Study the drawing (mm; zero at the part's minimum x, y, z) and answer. Coordinates: 2 decimals unless noted, no trailing zeros. Order: outer loops, then holes, each group sorted by start corner. A loop starts at its lowest first (then second) coordinate and runs counter-clockwise, first axis right, second up.
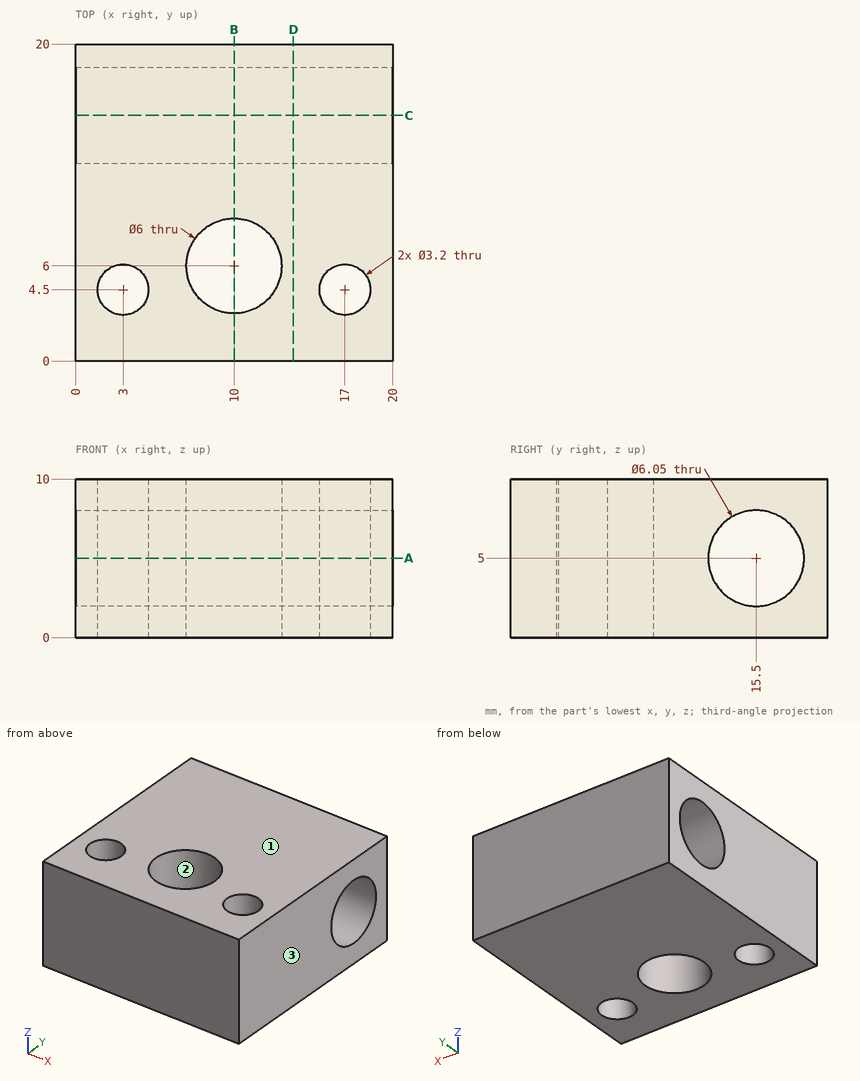
1) A flat-ended cylindrical pin translates along its axis: pin 1 Ø4 at (x, z) = (11.5, 4.5) entering from -Y. Find the tip coordinate at first contact, or state that the pin passes through.
A:
pin 1: stops at y = 0
2) A cutting plane is placed at A-A, the plane z = 5. Determine the outline of the cut face in (x, y) (3 decimals), and give its area (3 significant figures).
A:
outline: (0, 0) - (20, 0) - (20, 12.475) - (0, 12.475) - close; (0, 18.525) - (20, 18.525) - (20, 20) - (0, 20) - close; hole circle Ø3.2 at (3, 4.5); hole circle Ø6 at (10, 6); hole circle Ø3.2 at (17, 4.5)
area: 235 mm2
3) A cutting plane is placed at B-B, the plane x = 10. Determine the outline of the cut face in (y, z) (3 decimals), and give its area (3 significant figures).
A:
outline: (0, 0) - (3, 0) - (3, 10) - (0, 10) - close; (9, 0) - (20, 0) - (20, 10) - (9, 10) - close; hole circle Ø6.05 at (15.5, 5)
area: 111 mm2
4) A cutting plane is placed at D-D, the plane x = 13.75. Determine the outline of the cut face in (y, z) (3 decimals), and give its area (3 significant figures).
A:
outline: (0, 0) - (20, 0) - (20, 10) - (0, 10) - close; hole circle Ø6.05 at (15.5, 5)
area: 171 mm2
5) A cutting plane is placed at C-C, the plane y = 15.5. Determine the outline of the cut face in (x, z) (3 decimals).
A:
outline: (0, 0) - (20, 0) - (20, 1.975) - (0, 1.975) - close; (0, 8.025) - (20, 8.025) - (20, 10) - (0, 10) - close
6) Straight lines are drawn through the part: line 1 (Y direction, x = 3, z = 5) (3 decimals); line 2 (Y direction, x = 3, z = 2.75); line 3 (Y direction, x = 17, z = 8.25). For each, find the intervals that lie inside material, in ascending order.
A:
line 1: y = 0 to 2.9, 6.1 to 12.475, 18.525 to 20
line 2: y = 0 to 2.9, 6.1 to 13.48, 17.52 to 20
line 3: y = 0 to 2.9, 6.1 to 20
7) Determine the mould class of the marked faces 1, 2 and 3 for opening direction X: pulls with the +X half, pulls with the -X half, needs draft (parallel to the pull), parting line crosses it, or undercut.
A:
face 1: needs draft
face 2: undercut
face 3: pulls with the +X half
